Check sheet for the modelled part. Datum: model origin and axes. Units: mm. Face numbers are marked on the shaded views. A direction names the side the tool comes from. Give positions to 0.01 mm unless a question says otherwise; leave off trailing zeros. Order: outer loops, then holes, each group sorted by start corner. A loop starts at its lowest first (then second) coordinate and runs counter-clockwise, first axis right, second up.
from build123d import *

# Parameters (mm, degrees)
F1_DEPTH    = 20
F2_R        = 2.6
F3_DEPTH    = 50.6016350946
F4_COUNT    = 3
F4_ANGLE    = 240
F6_DEPTH    = 5
F7_T1_DEPTH = 25
F10_DEPTH   = 5
F11_DEPTH   = 25.001
F12_R       = 2
F13_R       = 2.6
F13_R_2     = 2.372590354
F14_DEPTH   = 25.001
F15_R       = 5
F16_R       = 4.5
F17_DEPTH   = 20


# Not quite as in the source:
# - a fillet or chamfer that OpenCascade refuses, or shapes differently, is made with other operations: its cross-section is extruded or revolved along the edge and cut away or added


with BuildPart() as f1:
    # F0 (on Top) → F1 (new body)
    with BuildSketch(Plane.XY):
        Polygon((43.0992290895, -36.5458269543), (6.7261621305, -15.5458269543), (16.8261621305, 1.9478862021), (53.1992290895, -19.0521137979), (55.6992290895, -14.7219867789), (14.8979589003, 8.8346375481), (0, 0), (-0.2020410997, -17.3193296462), (40.5992290895, -40.8759539732), align=None)
    extrude(amount=F1_DEPTH)

    # F2 (on face) → F3 (cut, through all)
    with BuildSketch(Plane(origin=(-7.55, -13.0769835971, 0), x_dir=(0.8660254038, -0.5, 0), z_dir=(-0.5, -0.8660254038, 0))):
        with Locations((45.5979407522, 10)):
            Circle(F2_R)
        with Locations((23.5979407522, 10)):
            Circle(F2_R)
    extrude(amount=-F3_DEPTH, mode=Mode.SUBTRACT)

    # F4: F1 ×3 about axis
    f4_axis = Axis((0, 0, 10), (0, 0, -1))


with BuildPart() as f1_1:
    add(f1.part)
    for i in range(1, F4_COUNT):
        add(f1.part.rotate(f4_axis, i * F4_ANGLE / (F4_COUNT - 1)))

    # F5 (on face) → F6 (join)
    with BuildSketch(Plane(origin=(0, 0, 0), x_dir=(1, 0, 0), z_dir=(0, 0, -1))):
        Polygon((0, 17.4359781295), (-40.5992290895, 40.8759539732), (-55.6992290895, 14.7219867789), (-15.1, -8.7179890648), (-15.1, -55.5979407522), (15.1, -55.5979407522), (15.1, -8.7179890648), (55.6992290895, 14.7219867789), (40.5992290895, 40.8759539732), align=None)
    extrude(amount=F6_DEPTH)

    # F7: fillet of radius 5 on 3 edges, made by hand

    # F7_s2 → F7_t1 (join)
    with BuildSketch(Plane.XY.offset(-5)):
        with BuildLine():
            ThreePointArc((2.5, -18.8792383324), (0, -18.2093653514), (-2.5, -18.8792383324))
            Line((-2.5, -18.8792383324), (-2.55, -18.7926357921))
            ThreePointArc((-2.55, -18.7926357921), (-1.299975, -18.0710489919), (-0.05, -17.3493755891))
            Line((-0.05, -17.3493755891), (0.05, -17.3493755891))
            ThreePointArc((0.05, -17.3493755891), (1.299975, -18.0710489919), (2.55, -18.7926357921))
            Line((2.55, -18.7926357921), (2.5, -18.8792383324))
        make_face()
        with BuildLine():
            ThreePointArc((15.0999, 11.6046826757), (15.7697729811, 9.1046826757), (17.5999, 7.2745556568))
            Line((17.5999, 7.2745556568), (17.5499, 7.1879531164))
            ThreePointArc((17.5499, 7.1879531164), (16.299975, 7.9097131217), (15.05, 8.6313865244))
            Line((15.05, 8.6313865244), (15, 8.7179890648))
            ThreePointArc((15, 8.7179890648), (15, 10.1613358702), (14.9999, 11.6046826757))
            Line((14.9999, 11.6046826757), (15.0999, 11.6046826757))
        make_face()
        with BuildLine():
            ThreePointArc((-17.5999, 7.2745556568), (-15.7697729811, 9.1046826757), (-15.0999, 11.6046826757))
            Line((-15.0999, 11.6046826757), (-14.9999, 11.6046826757))
            ThreePointArc((-14.9999, 11.6046826757), (-15, 10.1613358702), (-15, 8.7179890648))
            Line((-15, 8.7179890648), (-15.05, 8.6313865244))
            ThreePointArc((-15.05, 8.6313865244), (-16.299975, 7.9097131217), (-17.5499, 7.1879531164))
            Line((-17.5499, 7.1879531164), (-17.5999, 7.2745556568))
        make_face()
    extrude(amount=F7_T1_DEPTH)

    # F9 (on face) → F10 (join)
    with BuildSketch(Plane(origin=(0, 0, -5), x_dir=(1, 0, 0), z_dir=(0, 0, -1))):
        with BuildLine():
            Line((-55.6992290895, 14.7219867789), (-55.6992290895, -20))
            Line((-55.6992290895, -20), (55.6992290895, -20))
            Line((55.6992290895, -20), (55.6992290895, 14.7219867789))
            Line((55.6992290895, 14.7219867789), (52.6519667355, 20))
            Line((52.6519667355, 20), (4.4410161514, 20))
            Line((4.4410161514, 20), (2.5, 18.8793538025))
            ThreePointArc((2.5, 18.8793538025), (0, 18.2094808214), (-2.5, 18.8793538025))
            Line((-2.5, 18.8793538025), (-4.4410161514, 20))
            Line((-4.4410161514, 20), (-52.6519667355, 20))
            Line((-52.6519667355, 20), (-55.6992290895, 14.7219867789))
        make_face()
    extrude(amount=-F10_DEPTH)

    # F8 (on face) → F11 (cut, through all)
    with BuildSketch(Plane.XY.offset(20)):
        Polygon((10, 5.0614941438), (-10, 5.0614941438), (0, -12.2590139319), align=None)
    extrude(amount=-F11_DEPTH, mode=Mode.SUBTRACT)

    # F12
    f12_edges = [f1_1.edges().sort_by_distance(p)[0] for p in [
        (10, 5.061494, 7.5),
        (-10, 5.061494, 7.5),
        (0, -12.259014, 7.5),
    ]]
    fillet(f12_edges, radius=F12_R)

    # F13 (on face) → F14 (cut, through all)
    with BuildSketch(Plane(origin=(0, 0, -5), x_dir=(1, 0, 0), z_dir=(0, 0, -1))):
        with Locations((-40, -10)):
            Circle(F13_R)
        with Locations((40, -10)):
            Circle(F13_R_2)
        with Locations((0, 10)):
            Circle(F13_R)
    extrude(amount=-F14_DEPTH, mode=Mode.SUBTRACT)

    # F15
    f15_edges = [f1_1.edges().sort_by_distance(p)[0] for p in [
        (-15.1, 20, -2.5),
        (15.1, 20, -2.5),
        (55.699229, 20, -2.5),
        (-55.699229, 20, -2.5),
        (-12.6, 55.597941, 20),
        (12.6, 55.597941, 20),
        (-54.449229, -16.88705, 20),
        (-41.849229, -38.71089, 20),
        (54.449229, -16.88705, 20),
        (41.849229, -38.71089, 20),
    ]]
    fillet(f15_edges, radius=F15_R)

    # F16 (on face) → F17 (cut)
    with BuildSketch(Plane.XY.offset(20)):
        with Locations((0, -10)):
            Circle(F16_R)
    extrude(amount=-F17_DEPTH, mode=Mode.SUBTRACT)


solid = f1_1.part
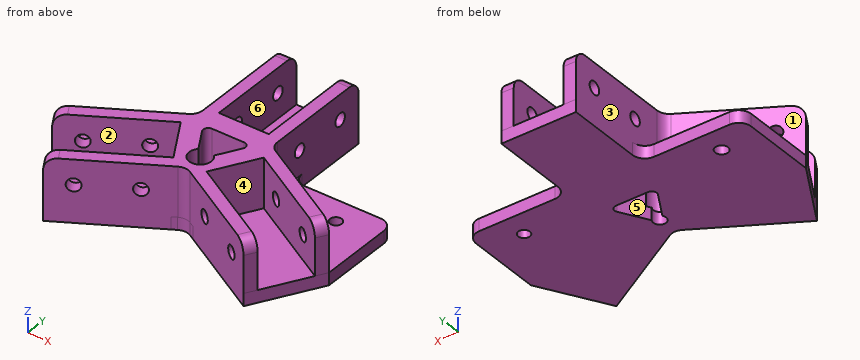
1) Section check B-B, the plane y = 29. Record the cut outline in (x, z), then the cut area to 3 significant figures.
Recorded:
outline: (-15.1, -5) - (15.1, -5) - (15.1, 20) - (10.1, 20) - (10.1, 0) - (-10.1, 0) - (-10.1, 20) - (-15.1, 20) - close
area: 351 mm2
2) Section check A-A, the plane y = 10. Record the cut outline in (x, z).
Recorded:
outline: (-55.7, -5) - (-42.6, -5) - (-42.6, 0) - (-55.7, 0) - close; (-37.4, -5) - (37.63, -5) - (37.63, 0) - (15.36, 0) - (15.36, 20) - (-15.36, 20) - (-15.36, 0) - (-37.4, 0) - close; (42.37, -5) - (55.7, -5) - (55.7, 0) - (42.37, 0) - close
3) Section check D-D, the plane x = -22. Record the cut outline in (y, z), then the cut area to 3 significant figures.
Recorded:
outline: (-30.14, -5) - (20, -5) - (20, 0) - (4.73, 0) - (4.73, 20) - (-1.04, 20) - (-1.04, 0) - (-24.36, 0) - (-24.36, 20) - (-30.14, 20) - close
area: 482 mm2
4) Depth check by flat-ended pin: pin 1 Ø3 at (y, z) = (45.6, 10) entering from -X; pin 2 Ø1 at (y, z) = (21, 3.5) entering from -X; pin 3 Ø4 at (x, z) = (29, 15.5) entering from +Y; pin 4 Ø10 at (x, z) = (-14.5, 2) entering from -Y. Enter the tip coordinate at first touch or a pass-through.
Recorded:
pin 1: passes through
pin 2: stops at x = -15.1
pin 3: stops at y = 1.85
pin 4: stops at y = -28.69
5) Set-up check for the marked faces 4, 5 and 6: record each of +Z, -Z, +X, -X, +Y, -Y from which the full face is reachable in a straight line by a thin tool's end or side.
Recorded:
face 4: +Z
face 5: +Z, -Z
face 6: +Z, +Y
6) Material ranges on L1, parallel to X at y = 10, z = -2.65; L2, parallel to X at y = 29.5, z = 17; L3, parallel to X at y = -1, z = 15.25, recorded low to high.
Recorded:
L1: x = -55.7 to -42.6, -37.4 to 37.63, 42.37 to 55.7
L2: x = -15.1 to -10.1, 10.1 to 15.1
L3: x = -31.93 to -21.93, -15.12 to -6.5, 6.5 to 15.12, 21.93 to 31.93
7) Draft check along Y on the marked faces 1, 2 and 3. Enter one of: +Y half, -Y half, draft (parallel to the pull), parting line (faces both ways), or undercut.
Recorded:
face 1: +Y half
face 2: undercut
face 3: draft
